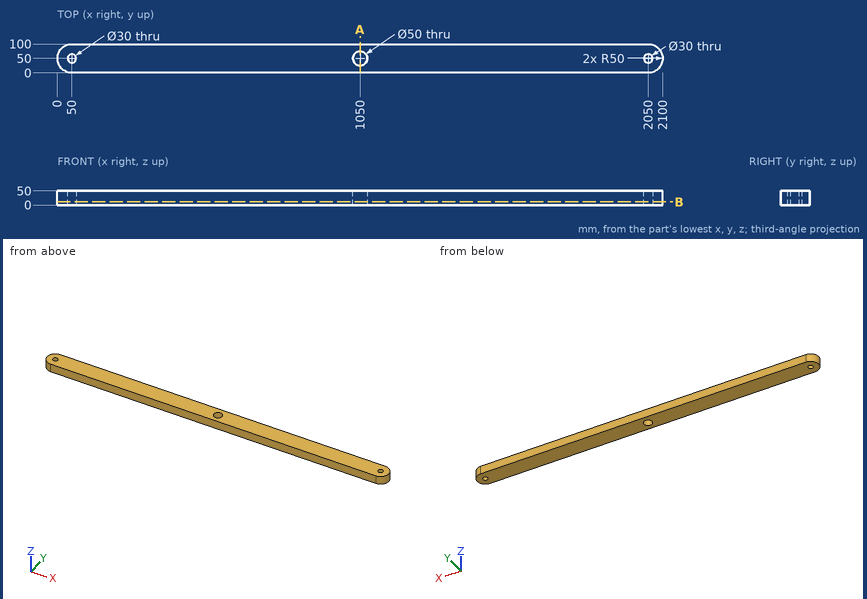
Check sheet for the drawn part. Datum: minimum x, y, z corner. Units: mm. Give positions to 0.01 mm unless a question says otherwise; leave off trailing zeros. Loops run counter-clockwise (first coordinate to the right, second up) from the corner with the lowest first, then second, coordinate; pieces in that order, holes last.
1) Sectioned sample at B-B, the plane z = 12. Enter the section's corners in (x, y).
2) Sectioned sample at A-A, the plane x = 1050. Enter the section's corners in (y, z).
3) Depth check by flat-ended pin: pin 1 Ø5 at (y, z) = (35, 33.5) entering from -X; pin 2 Ø5 at (y, z) = (16, 17) entering from +X; pin 3 Ø2 at (y, z) = (38, 20.5) entering from -X (3 decimals). Enter the tip coordinate at first touch or a pass-through.
4) Thickness scan on line 1 along Y through (x, z) = (50, 16); line 2 along X through (y, z) = (54.5, 32.5); line 3 along X through (y, z) = (60.5, 44). Record the ranges inside material, lowest first.
Answers:
1. outline: (50, 0) - (2050, 0) arc R50 ccw to (2050, 100) - (50, 100) arc R50 ccw to start; hole circle Ø30 at (50, 50); hole circle Ø50 at (1050, 50); hole circle Ø30 at (2050, 50)
2. outline: (0, 0) - (25, 0) - (25, 50) - (0, 50) - close; (75, 0) - (100, 0) - (100, 50) - (75, 50) - close
3. pin 1: stops at x = 1.59
3. pin 2: stops at x = 2088.83
3. pin 3: stops at x = 1.225
4. line 1: y = 0 to 35, 65 to 100
4. line 2: x = 0.2 to 35.69, 64.31 to 1025.41, 1074.59 to 2035.69, 2064.31 to 2099.8
4. line 3: x = 1.11 to 39.29, 60.71 to 1027.31, 1072.69 to 2039.29, 2060.71 to 2098.89
